```python
from build123d import *

# Parameters (mm, degrees)
SKETCH_1_R      = 1.05
EXTRUDE_1_DEPTH = 2
SKETCH_2_W      = 3
SKETCH_2_H      = 3
EXTRUDE_2_DEPTH = 1


with BuildPart() as part:
    # 草图1 → 凸台-拉伸1 (new body)
    with BuildSketch(Plane(origin=(0, 0, 0), x_dir=(1, 0, 0), z_dir=(0, 1, 0))):
        with BuildLine():
            Line((1, 0), (22, 0))
            ThreePointArc((22, 0), (22.707106781, 0.292893219), (23, 1))
            Line((23, 1), (23, 14))
            ThreePointArc((23, 14), (22.707106781, 14.707106781), (22, 15))
            Line((22, 15), (1, 15))
            ThreePointArc((1, 15), (0.292893219, 14.707106781), (0, 14))
            Line((0, 14), (0, 1))
            ThreePointArc((0, 1), (0.292893219, 0.292893219), (1, 0))
        make_face()
        with Locations(Location((2.5, 2.5, 0), (0, 0, 270))):
            Circle(SKETCH_1_R, mode=Mode.SUBTRACT)
        with Locations(Location((20.5, 2.5, 0), (0, 0, 90))):
            Circle(SKETCH_1_R, mode=Mode.SUBTRACT)
    extrude(amount=EXTRUDE_1_DEPTH)

    # 草图2 → 凸台-拉伸2 (add)
    with BuildSketch(Plane(origin=(0, 2, 0), x_dir=(1, 0, 0), z_dir=(0, 1, 0))):
        with Locations((10.5, 4.160508355)):
            Rectangle(SKETCH_2_W, SKETCH_2_H)
    extrude(amount=EXTRUDE_2_DEPTH)


solid = part.part
```
Geometry check sheet. Reference: the model listing, model coordinates, mm. A direction names the side the tool comes from. Give positions to 0.01 mm unless a question says otherwise; leave off trailing zeros. Order: outer loops, then holes, each group sorted by start corner. A loop starts at its lowest first (then second) coordinate and runs counter-clockwise, first axis right, second up. Notation, with made-up numbers: (-19.5, 67.5) - (37.5, 67.5) arc R19 cw to (37.5, 85.5) - close; hole circle Ø10 at (-5.75, 11.25). An arc over 180 degrees is marked (long way). Write item = value, one per line. Start each with the question number.
1) Access from +Z, -Z, +X, -X, +Y, -Y to the whole of each face (thin tool, end or side, straight path). Record for faces 1 (the flat face through (10.5, 2.5, -5.661)), 2 (the flat face through (9, 2.5, -4.1)), 3 (the flat face through (10.5, 2.5, -2.661)), 4 (the flat face through (12, 2.5, -4.1)).
2) Section check D-D (z = -6). Enter the section's corners in (x, y).
3) Gauge pin test, flat ends, axial feed: pin 1 Ø1.7 at (x, z) = (2.5, -2.5) entering from -Y; pin 2 Ø0.8 at (y, z) = (2.5, -4.5) entering from -X; pin 3 Ø0.5 at (y, z) = (2.5, -3.5) entering from +X. Record the tip position at first contact, or that the pin passes through.
4) Section check C-C (y = 2.25). Enter the section's corners in (x, z), then the cut area to 3 significant figures.
5) Scan lines: L1, parallel to X at y = 1.6, z = -2.5; L2, parallel to X at y = 0.3, z = -2; L3, parallel to Z at x = 20.5, y = 0.4. Record each from-to range of solid material in increasing order.
6) Section check A-A (x = 20.5). Enter the section's corners in (y, z).
7) Section check B-B (y = 0.5). Enter the section's corners in (x, z), then the cut area to 3 significant figures.
Geometry check:
q1.face_1 = -Z, +X, -X, +Y
q1.face_2 = +Z, -Z, -X, +Y
q1.face_3 = +Z, +X, -X, +Y
q1.face_4 = +Z, -Z, +X, +Y
q2.outline = (0, 0) - (23, 0) - (23, 2) - (0, 2) - close
q3.pin_1 = through
q3.pin_2 = 9
q3.pin_3 = 12
q4.outline = (9, -5.66) - (12, -5.66) - (12, -2.66) - (9, -2.66) - close
q4.area = 9.00 mm2
q5.L1 = 0 to 1.45, 3.55 to 19.45, 21.55 to 23
q5.L2 = 0 to 1.58, 3.42 to 19.58, 21.42 to 23
q5.L3 = -15 to -3.55, -1.45 to 0
q6.outline = (0, -15) - (2, -15) - (2, -3.55) - (0, -3.55) - close; (0, -1.45) - (2, -1.45) - (2, 0) - (0, 0) - close
q7.outline = (0, -14) arc R1 ccw to (1, -15) - (22, -15) arc R1 ccw to (23, -14) - (23, -1) arc R1 ccw to (22, 0) - (1, 0) arc R1 ccw to (0, -1) - close; hole circle Ø2.1 at (2.5, -2.5); hole circle Ø2.1 at (20.5, -2.5)
q7.area = 337 mm2
